```python
from build123d import *

# Parameters (mm, degrees)
F0_R     = 1.6
F1_DEPTH = 0.9


with BuildPart() as f1:
    # F0 (on Top) → F1 (new body)
    with BuildSketch(Plane.XY):
        Polygon((-23.225, -14.8725), (-22.325, -15.7725), (23.225, -15.7725), (23.225, 14.7725), (22.225, 15.7725), (-3.783311, 15.7725), (-11.325, 8.3275), (-16.165, 8.3275), (-17.675, 6.8275), (-17.675, 1.3675), (-22.235, 1.3775), (-23.225, 0.3875), (-23.225, -7.3323), (-23.225, -13.0127), align=None)
        with Locations((-15.225, -13.2725)):
            Circle(F0_R, mode=Mode.SUBTRACT)
        with Locations((4.025, -13.2725)):
            Circle(F0_R, mode=Mode.SUBTRACT)
        with Locations((17.125, -13.2725)):
            Circle(F0_R, mode=Mode.SUBTRACT)
        with Locations((-15.025, 5.627501)):
            Circle(F0_R, mode=Mode.SUBTRACT)
        with Locations((-4.575, 0.2275)):
            Circle(F0_R, mode=Mode.SUBTRACT)
        with Locations((17.125, 0.0275)):
            Circle(F0_R, mode=Mode.SUBTRACT)
        with Locations((4.025, 12.6275)):
            Circle(F0_R, mode=Mode.SUBTRACT)
        with Locations((17.125, 12.6275)):
            Circle(F0_R, mode=Mode.SUBTRACT)
    extrude(amount=F1_DEPTH)


solid = f1.part
```
Work out the finished part from the listing and answer in its coordinate system (mm). A direction names the side the tool comes from. Give positions to 0.01 mm unless a question says otherwise; leave off trailing zeros. Order: outer loops, then holes, each group sorted by start corner. A loop starts at its lowest first (then second) coordinate and runs counter-clockwise, first axis right, second up. Notation, with made-up numbers: (50, -27) -> (82, -27) arc R30 ccw to (82, -3) -> close; hole circle Ø2 at (83, -25). An arc over 180 degrees is marked (long way). Answer as CSV lines item,"result". Start each with the question number.
(1) This flat-tipped pin is pushed along its axis until it touches: pin 1 Ø2.5 at (x, y) = (-15.02, 5.63) entering from +Z. Where does it stop, or does it pass through?
(2) Section B-B, the plane z = 0.4 is taken. Give the number of separate pieces and of enclosed holes in the cut face, plus the area to 3 significant figures.
(3) For a pull along X with two mould halves and no side action, classify faces 3 (the flat face through (22.7, 15.3, 0.4)), 4 (the flat face through (-13.7, 8.328, 0.4)), 5 (the flat face through (-7.501, 12.102, 0.444)), 6 (the cylindrical face through (15.527, 0.098, 0.444)) as released by +X, released by -X, zero draft, split by the parting line, or undercut.
(4) Section D-D, the plane x = 16 is taken. Write down the section's boundary in (y, z).
(5) Consider line 1 along Y through (x, z) = (18, 0.65); line 2 along Y through (x, z) = (5, 0.55); line 3 along Y through (x, z) = (-16, 0.55). Determine where each line is inside the solid, lowest interval first.
(6) Section C-C, the plane x = -4.5 is taken. Write down the section's boundary in (y, z) (1 decimal).
(7) Which of the six approach directions +Z, -Z, +X, -X, +Y, -Y give full straight-line access (tool end or side, diameter ignored) to faces 1 (the flat face through (-17.675, 4.1, 0.4)), 2 (the flat face through (9.4, 15.772, 0.4))?
(8) Section A-A, the plane y = 11.5 is taken. Write down the section's boundary in (x, z) (3 decimals), plus the area to 3 significant figures.
Entries:
1,pin 1,"through"
2,separate pieces,"1"
2,enclosed holes,"8"
2,area,"1,240 mm²"
3,face 3,"released by +X"
3,face 4,"zero draft"
3,face 5,"released by -X"
3,face 6,"undercut"
4,outline,"(-15.77, 0) -> (-14.41, 0) -> (-14.41, 0.9) -> (-15.77, 0.9) -> close; (-12.13, 0) -> (-1.11, 0) -> (-1.11, 0.9) -> (-12.13, 0.9) -> close; (1.17, 0) -> (11.49, 0) -> (11.49, 0.9) -> (1.17, 0.9) -> close; (13.77, 0) -> (15.77, 0) -> (15.77, 0.9) -> (13.77, 0.9) -> close"
5,line 1,"-15.77 to -14.61, -11.93 to -1.31, 1.37 to 11.29, 13.97 to 15.77"
5,line 2,"-15.77 to -14.54, -12 to 11.36, 13.9 to 15.77"
5,line 3,"-15.77 to -14.67, -11.87 to 4.36, 6.9 to 8.33"
6,outline,"(-15.8, 0) -> (-1.4, 0) -> (-1.4, 0.9) -> (-15.8, 0.9) -> close; (1.8, 0) -> (15.1, 0) -> (15.1, 0.9) -> (1.8, 0.9) -> close"
7,face 1,"+Z, -Z, -X, +Y"
7,face 2,"+Z, -Z, +X, -X, +Y"
8,outline,"(-8.111, 0) -> (2.89, 0) -> (2.89, 0.9) -> (-8.111, 0.9) -> close; (5.16, 0) -> (15.99, 0) -> (15.99, 0.9) -> (5.16, 0.9) -> close; (18.26, 0) -> (23.225, 0) -> (23.225, 0.9) -> (18.26, 0.9) -> close"
8,area,"24.1 mm²"
